The model under review builds one solid part; all positions refer to its coordinate system, in mm. A direction names the side the tool comes from. Round coordinates to 2 decimals unless told otherwise and drop trailing zeros. Write each loop counter-clockwise with the first axis right and the second up, starting at its lowest first coordinate (ties: lowest second). Pieces come first, ordered by that corner, then holes. Notation, with made-up numbers: M 23,74 L 67,74 A32 cw 67,113 Z; hole C 60,60.5 d7. An arc over 180 degrees is marked long. One line per item, written item: value. Start each with the question number.
1) Take a section at D-D, the plane y = 48.5. Write out the cut boundary in (x, z), and give its area (3 significant figures).
2) Take a section at C-C, the plane z = -12. Write out the cut boundary in (x, y).
3) Take a section at A-A, the plane y = 37. Write out the cut boundary in (x, z), and give its area (3 significant figures).
4) Take a section at B-B, the plane z = -30. Write out the cut boundary in (x, y), and give its area (3 significant figures).
5) Mouldability with a two-part tool opening along Z and no side actions: class faces 1 (the face through (3.944, 2.333, -31.97)), 2 (the face through (4.958, 49.126, -33.795)), 3 (the face through (3.944, 17.943, -36.678)) as +Z half, -Z half, draft (parallel to the pull), parting line (faces both ways), or undercut.
6) Wall thickness on probe 1 along X at (y, z) = (44, -30.75); probe 2 along Y at (x, z) = (2.5, -31); probe 3 along X at (y, z) = (56, -19.5): over which ranges is each line inside the solid? List them lowest first.
7) Tool access review of faces 4 (the face through (1, 43.9, -36.6)), 5 (the face through (3.94, 53.72, -11.97)), 6 (the face through (4.84, 33.24, -32.28)), 7 (the face through (0, 30, -23)), 8 (the face through (5, 37.1, -6.8)): name each direction out of +Z, -Z, +X, -X, +Y, -Y from which nothing blocks a thin tool from reaching the whole face with its end or side.
8) For P1, Ø3, axis at x = 4.5, z = -19, coming from the -Y side; P2, Ø1, axis at x = 5, y = 57, coming from the +Z side; P3, Ø3, axis at x = 5, y = 44, coming from the +Z side, all flat-tipped, find the tip position at first contact; note any pin that passes through.
from build123d import *

# Parameters (mm, degrees)
SKETCH27_R                  = 3.55
SKETCH27_R_2                = 5
SKETCH27_R_3                = 2.5
BOSS_EXTRUDE1_DEPTH         = 8
TAP_DRILL_FOR_M3_TAP2_D     = 2.5
TAP_DRILL_FOR_M3_TAP2_DEPTH = 10
TAP_DRILL_FOR_M3_TAP2_TIP   = 0.751075774
SKETCH47_R                  = 7.99
CUT_EXTRUDE8_DEPTH          = 5
CUT_EXTRUDE10_DEPTH         = 2
CUT_EXTRUDE11_REACH         = 78.755
SKETCH49_R                  = 1.5


with BuildPart() as part:
    # Sketch27 → Boss-Extrude1 (new body)
    with BuildSketch(Plane(origin=(0, 0, 0), x_dir=(0, 0, -1), z_dir=(1, 0, 0))):
        with BuildLine():
            Line((3.703427373, 44.222664512), (20.469158548, 63.481222917))
            ThreePointArc((20.469158548, 63.481222917), (31.099959488, 66.174951681), (37.349351573, 57.163003953))
            Line((37.349351573, 57.163003953), (37.349351573, 28))
            Line((37.349351573, 28), (35.98665831, 7.600097167))
            ThreePointArc((35.98665831, 7.600097167), (31.875470614, 2.300648285), (25.420672816, 4.12317623))
            Line((25.420672816, 4.12317623), (3.604566829, 29.892489756))
            ThreePointArc((3.604566829, 29.892489756), (1.000261752, 37.075884637), (3.703427373, 44.222664512))
        make_face()
        with Locations((29.349351573, 55)):
            Circle(SKETCH27_R, mode=Mode.SUBTRACT)
        with Locations((12, 37)):
            Circle(SKETCH27_R_2, mode=Mode.SUBTRACT)
        with Locations((30, 8)):
            Circle(SKETCH27_R_3, mode=Mode.SUBTRACT)
    extrude(amount=BOSS_EXTRUDE1_DEPTH)

    # Tap Drill for M3 Tap2
    with Locations(Plane(origin=(0, 0, -37.349351573), x_dir=(-1, 0, 0), z_dir=(0, 0, -1))):
        with Locations((-5, 44), (-5, 32)):
            Hole(TAP_DRILL_FOR_M3_TAP2_D / 2, depth=TAP_DRILL_FOR_M3_TAP2_DEPTH)
            with Locations((0, 0, -(TAP_DRILL_FOR_M3_TAP2_DEPTH + TAP_DRILL_FOR_M3_TAP2_TIP / 2))):  # 118° drill point
                Cone(0, TAP_DRILL_FOR_M3_TAP2_D / 2, TAP_DRILL_FOR_M3_TAP2_TIP, mode=Mode.SUBTRACT)

    # Sketch47 → Cut-Extrude8 (cut)
    with BuildSketch(Plane.ZY):
        with Locations((-12, 37)):
            Circle(SKETCH47_R)
    extrude(amount=-CUT_EXTRUDE8_DEPTH, mode=Mode.SUBTRACT)

    # Sketch48 → Cut-Extrude10 (cut)
    with BuildSketch(Plane.ZY):
        with BuildLine():
            Line((-37.349351573, 42.600403232), (-37.349351573, 72.646655563))
            Line((-37.349351573, 72.646655563), (-14.22165601, 72.646655563))
            Line((-14.22165601, 72.646655563), (-14.22165601, 56.304805064))
            ThreePointArc((-14.22165601, 56.304805064), (-15.894843611, 56.718614571), (-16.852615188, 55.285621667))
            ThreePointArc((-16.852615188, 55.285621667), (-22.758204677, 44.378946258), (-35.152923001, 43.928931457))
            ThreePointArc((-35.152923001, 43.928931457), (-36.625675327, 43.883883434), (-37.349351573, 42.600403232))
        make_face()
    extrude(amount=-CUT_EXTRUDE10_DEPTH, mode=Mode.SUBTRACT)

    # Sketch49 → Cut-Extrude11 (cut, up to next)
    with BuildSketch(Plane.ZY.offset(-2), mode=Mode.PRIVATE) as cut_extrude11_sk1:
        with Locations((-33.599351573, 47.638784068)):
            Circle(SKETCH49_R)
    cut_extrude11_tool1 = extrude(cut_extrude11_sk1.sketch, amount=-CUT_EXTRUDE11_REACH, mode=Mode.PRIVATE) & part.part
    # Sketch49 → Cut-Extrude11 (cut, up to next)
    with BuildSketch(Plane.ZY.offset(-2), mode=Mode.PRIVATE) as cut_extrude11_sk2:
        with Locations((-25.099351573, 62.361215932)):
            Circle(SKETCH49_R)
    cut_extrude11_tool2 = extrude(cut_extrude11_sk2.sketch, amount=-CUT_EXTRUDE11_REACH, mode=Mode.PRIVATE) & part.part
    add(cut_extrude11_tool1.solids().sort_by_distance((2, 47.638784, -33.599352))[0], mode=Mode.SUBTRACT)
    add(cut_extrude11_tool2.solids().sort_by_distance((2, 62.361216, -25.099352))[0], mode=Mode.SUBTRACT)


solid = part.part
Checked values:
1. outline: M 0,-18.67 L 2,-18.67 L 2,-32.37 L 8,-32.37 L 8,-7.43 L 0,-7.43 Z; M 2,-37.35 L 8,-37.35 L 8,-34.83 L 2,-34.83 Z
1. area: 187 mm2
2. outline: M 0,19.98 L 8,19.98 L 8,32 L 5,32 L 5,29.01 L 0,29.01 Z; M 0,44.99 L 5,44.99 L 5,42 L 8,42 L 8,53.75 L 0,53.75 Z
3. outline: M 0,-37.35 L 8,-37.35 L 8,-17 L 5,-17 L 5,-19.99 L 0,-19.99 Z; M 0,-4.01 L 5,-4.01 L 5,-7 L 8,-7 L 8,-1 L 0,-1 Z
3. area: 181 mm2
4. outline: M 0,2 L 8,2 L 8,5.5 L 0,5.5 Z; M 0,10.5 L 8,10.5 L 8,51.51 L 2,51.51 L 2,42.52 L 0,42.52 Z; M 2,58.49 L 8,58.49 L 8,66.51 L 2,66.51 Z; hole C 5,32 d2.5; hole C 5,44 d2.5
4. area: 376 mm2
5. face 1: parting line
5. face 2: undercut
5. face 3: -Z half
6. probe 1: x = 2 to 3.75, 6.25 to 8
6. probe 2: y = 2.08 to 5.71, 10.29 to 51.86, 58.14 to 66.21
6. probe 3: x = 2 to 8
7. face 4: -X, +Y
7. face 5: +Z, +X, -X, +Y
7. face 6: -Z
7. face 7: +Z, -Z, -X, +Y, -Y
7. face 8: -X
8. P1: stops at y = 9.94
8. P2: stops at z = -14.39
8. P3: stops at z = -2.47
